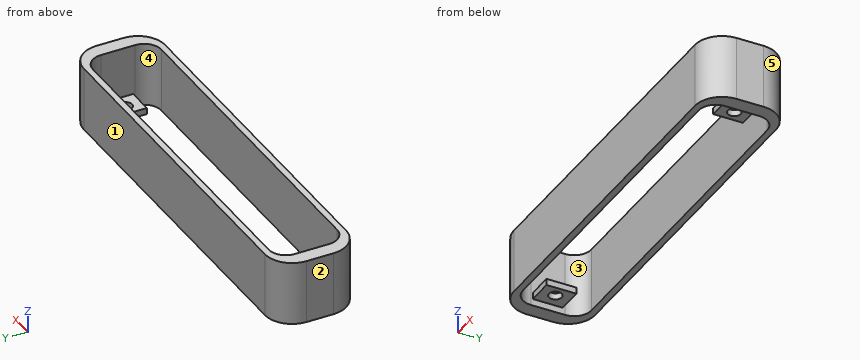
from build123d import *

# Parameters (mm, degrees)
SKETCH001_W   = 92
SKETCH001_H   = 18.98
SKETCH001_W_2 = 85
SKETCH001_H_2 = 15.98
PAD001_DEPTH  = 15
FILLET001_R   = 4
FILLET002_R   = 6.35
SKETCH080_W   = 7
SKETCH080_H   = 1.5
PAD002_DEPTH  = 6
SKETCH081_W   = 7
SKETCH081_H   = 1.5
PAD003_DEPTH  = 6
SKETCH082_R   = 1.5
POCKET_DEPTH  = 5


with BuildPart() as part:
    # Sketch001 → Pad001 (new body)
    with BuildSketch(Plane.XY):
        with Locations((47, -48.990001)):
            Rectangle(SKETCH001_W, SKETCH001_H)
        with Locations((47, -48.990001)):
            Rectangle(SKETCH001_W_2, SKETCH001_H_2, mode=Mode.SUBTRACT)
    extrude(amount=PAD001_DEPTH)

    # Fillet001
    fillet001_edges = [part.edges().sort_by_distance(p)[0] for p in [
        (4.5, -41.000001, 7.5),
        (89.5, -41.000001, 7.5),
        (89.5, -56.980001, 7.5),
        (4.5, -56.980001, 7.5),
    ]]
    fillet(fillet001_edges, radius=FILLET001_R)

    # Fillet002
    fillet002_edges = [part.edges().sort_by_distance(p)[0] for p in [
        (1, -39.500001, 7.5),
        (1, -58.480001, 7.5),
        (93, -39.500001, 7.5),
        (93, -58.480001, 7.5),
    ]]
    fillet(fillet002_edges, radius=FILLET002_R)

    # Sketch080 (on Face13 of Fillet002) → Pad002 (join)
    with BuildSketch(Plane(origin=(89.5, 0, 0), x_dir=(0, -1, 0), z_dir=(-1, 0, 0))):
        with Locations((49.039999, 2.35)):
            Rectangle(SKETCH080_W, SKETCH080_H)
    extrude(amount=PAD002_DEPTH)

    # Sketch081 (on Face14 of Pad002) → Pad003 (join)
    with BuildSketch(Plane.YZ.offset(4.5)):
        with Locations((-49.039999, 2.35)):
            Rectangle(SKETCH081_W, SKETCH081_H)
    extrude(amount=PAD003_DEPTH)

    # Sketch082 (on Face1 of Pad003) → Pocket (cut)
    with BuildSketch(Plane(origin=(0, 0, 0), x_dir=(1, 0, 0), z_dir=(0, 0, -1))):
        with Locations((7.84, 49.039999)):
            Circle(SKETCH082_R)
        with Locations((86.180001, 49.039999)):
            Circle(SKETCH082_R)
    extrude(amount=-POCKET_DEPTH, mode=Mode.SUBTRACT)


solid = part.part
Verification items for the finished model (mm, model axes). Face numbers are marked on the shaded views. A direction names the side the tool comes from. Round coordinates to 2 decimals unless told otherwise and drop trailing zeros. Loops run counter-clockwise (first coordinate to the right, second up) from the corner with the lowest first, then second, coordinate; pieces in that order, holes last. Notation, with made-up numbers: (19.5, 61.25) - (23.5, 61.25) arc R10 cw to (23.5, 74.25) - close; hole circle Ø3 at (-5, 20). An arc over 180 degrees is marked (long way). Use a Markdown table: item, result. Add a question column.
1. Thickness scan on probe 1 along X at (y, z) = (-46, 7); probe 2 along Y at (x, z) = (43, 3.75); probe 3 along Y at (x, z) = (88, 1.75). Record the ranges inside material, lowest first. Write a range as [from, to].
2. Section check A-A, the plane y = -49.04. Record the boundary of the cut face in (x, z).
3. Release check for a two-part mould opening along X. For the marked faces 1, 2 and 3 record: released by +X, released by -X, zero draft, split by the parting line, or undercut.
4. Section check B-B, the plane x = 65. Record the boundary of the cut face in (y, z).
5. Gauge pin test, flat ends, axial feed: pin 1 (3 mm diameter, centred on x = 7, y = -50.5, fed in from +Z); pin 2 (5 mm diameter, centred on x = 7.84, y = -49.04, fed in from -Z); pin 3 (1.2 mm diameter, centred on x = 6, z = 2.5, fed in from -Y). Record the tip position at first contact, or that the pin passes through.
6. Section check C-C, the plane z = 10.5. Record the boundary of the cut face in (x, y).
7. Access from +Z, -Z, +X, -X, +Y, -Y to the whole of each face (thin tool, end or side, straight path). Record for the marked faces 4 and 5.
Checks:
| question | item | result |
|---|---|---|
| 1 | probe 1 | x = [1, 4.5], [89.5, 93] |
| 1 | probe 2 | y = [-58.48, -56.98], [-41, -39.5] |
| 1 | probe 3 | y = [-58.33, -56.1], [-52.54, -45.54], [-41.88, -39.65] |
| 2 | outline | (1, 0) - (4.5, 0) - (4.5, 1.6) - (6.34, 1.6) - (6.34, 3.1) - (4.5, 3.1) - (4.5, 15) - (1, 15) - close; (9.34, 1.6) - (10.5, 1.6) - (10.5, 3.1) - (9.34, 3.1) - close; (83.5, 1.6) - (84.68, 1.6) - (84.68, 3.1) - (83.5, 3.1) - close; (87.68, 1.6) - (89.5, 1.6) - (89.5, 0) - (93, 0) - (93, 15) - (89.5, 15) - (89.5, 3.1) - (87.68, 3.1) - close |
| 3 | face 1 | zero draft |
| 3 | face 2 | released by -X |
| 3 | face 3 | undercut |
| 4 | outline | (-58.48, 0) - (-56.98, 0) - (-56.98, 15) - (-58.48, 15) - close; (-41, 0) - (-39.5, 0) - (-39.5, 15) - (-41, 15) - close |
| 5 | pin 1 | stops at z = 3.1 |
| 5 | pin 2 | stops at z = 1.6 |
| 5 | pin 3 | stops at y = -58.44 |
| 6 | outline | (1, -52.13) arc R6.35 ccw to (7.35, -58.48) - (86.65, -58.48) arc R6.35 ccw to (93, -52.13) - (93, -45.85) arc R6.35 ccw to (86.65, -39.5) - (7.35, -39.5) arc R6.35 ccw to (1, -45.85) - close; hole (4.5, -52.98) arc R4 ccw to (8.5, -56.98) - (85.5, -56.98) arc R4 ccw to (89.5, -52.98) - (89.5, -45) arc R4 ccw to (85.5, -41) - (8.5, -41) arc R4 ccw to (4.5, -45) - close |
| 7 | face 4 | +Z, -Z |
| 7 | face 5 | +Z, -Z, +X, +Y |
